Part model, mm, in its own coordinate system. A direction names the side the tool comes from. Round coordinates to 2 decimals unless told otherwise and drop trailing zeros. Write each loop counter-clockwise with the first axis right and the second up, starting at its lowest first coordinate (ties: lowest second). Pieces come first, ordered by that corner, then holes. Notation, with made-up numbers: M 30,-18 L 48,-18 A17 cw 48,-6 Z; hole C 44.25,59.5 d5. An arc over 180 degrees is marked long. Use a Markdown table: item, result. Add a question column.
1) Slice it at B-B on z = 59.5. Write the cut outline in (x, y), plus the area to 3 significant figures.
2) Two-plate mould, pull along X, no slides. Class faces 3 (the face through (-7, 18, 0)), 4 (the face through (-500, -18, 49)), 5 (the face through (500, 18, 49)), 6 (the face through (-416, 18, 100)): released by +X, released by -X, zero draft, split by the parting line, or undercut.
3) Which spindle directions (+Z, -Z, +X, -X, +Y, -Y) get a long thin tool onto all of the face, cutting with end or side? Do faces 1 (the face through (331, 18, 100)), 2 (the face through (77, -1300, 53)). Say none if no direction does.
4) Slice it at C-C on x = -426.5. Write the cut outline in (y, z).
5) Drop flat-ended pins along their axis: P1, Ø4, axis at x = 28.5, y = 896, coming from the -Z side; P2, Ø2, axis at x = -5.5, y = 582, coming from the +Z side; P3, Ø5, axis at y = 63.5, z = 106.5, coming from the +X side; P4, Ø12, axis at x = 215.5, y = -258.5, coming from the +Z side. Give the stop position or say it passes through.
6) Slice it at A-A on y = 389. Write the cut outline in (x, z).
7) Wall check: probe 1 along X at (y, z) = (-9, 125); probe 2 along X at (y, z) = (606, 11); probe 3 along X at (y, z) = (547, 133.5). Give the ranges that are in metal, low to high.
Autodesk Inventor part; units mm, degrees
ref_plane "YZ Plane" through (0, 0, 0) normal (1, 0, 0) x (0, 1, 0)
ref_plane "XZ Plane" through (0, 0, 0) normal (0, 1, 0) x (-1, 0, 0)
ref_plane "XY Plane" through (0, 0, 0) normal (0, 0, 1) x (1, 0, 0)
sketch "Sketch1" plane through (0, 0, 0) normal (0, 0, 1) x (1, 0, 0)
  line L0 (-500, 1300) -> (500, 1300)
  line L1 (500, 1300) -> (500, -1300)
  line L2 (500, -1300) -> (-500, -1300)
  line L3 (-500, -1300) -> (-500, 1300)
  line L4 (-500, 1300) -> (500, -1300) construction
  line L5 (500, 1300) -> (-500, -1300) construction
  point P0 (0, 0)
  dimension "d0" = 1000
  dimension "d1" = 2600
extrude "Extrusion1" add sketch "Sketch1" along normal blind 100
sketch "Sketch2" plane through (-500, -1300, 0) normal (0, -1, 0) x (1, 0, 0)
  line L0 (0, 0) -> (1000, 0)
  line L1 (1000, 0) -> (1000, 100)
  line L2 (0, 100) -> (1000, 100)
  line L3 (0, 0) -> (0, 100)
  line L4 (0, 100) -> (1000, 100)
  line L5 (1000, 100) -> (977, 135)
  line L6 (977, 135) -> (937, 135)
  line L7 (937, 135) -> (914, 100)
  line L8 (687, 135) -> (664, 100)
  line L9 (727, 135) -> (687, 135)
  line L10 (750, 100) -> (727, 135)
  line L11 (437, 135) -> (414, 100)
  line L12 (477, 135) -> (437, 135)
  line L13 (500, 100) -> (477, 135)
  line L14 (187, 135) -> (164, 100)
  line L15 (227, 135) -> (187, 135)
  line L16 (250, 100) -> (227, 135)
  line L17 (-63, 135) -> (-86, 100)
  line L18 (-23, 135) -> (-63, 135)
  line L19 (0, 100) -> (-23, 135)
  line L20 (-90.1785, 102.7459) -> (-65.6973, 140)
  line L21 (-65.6973, 140) -> (-20.3027, 140)
  line L22 (-20.3027, 140) -> (5.983, 100)
  line L23 (-90.1785, 102.7459) -> (-86, 100)
  point P0 (500, 0)
  point P1 (5.983, 100)
  dimension "d4" = 86
  dimension "d5" = 40
  dimension "d6" = 35
  dimension "d11" = 250
  dimension "d16" = 5
  dimension "d17" = 5
extrude "Extrusion2" add sketch "Sketch2" against normal up to surface (2600 mm away) contours L19 L18 L17 L23 L20 L21 L22 L2 | L2 L7 L6 L5 | L14 L15 L16 L2 | L2 L8 L9 L10 | L11 L12 L13 L2
chamfer "Chamfer1" distance 10 angle 45 2 edges at (500, -1300, 50) (500, 1300, 50)
equation "\"d17\" = d16"
properties part number "Sandwich 5  roof long"
Entries:
| question | item | result |
|---|---|---|
| 1 | outline | M -500,-1300 L 490,-1300 L 500,-1290 L 500,1290 L 490,1300 L -500,1300 Z |
| 1 | area | 2,600,000 mm^2 |
| 2 | face 3 | zero draft |
| 2 | face 4 | released by -X |
| 2 | face 5 | released by +X |
| 2 | face 6 | undercut |
| 3 | face 1 | +Z, +Y, -Y |
| 3 | face 2 | +Z, -Z, +X, -X, -Y |
| 4 | outline | M -1300,0 L 1300,0 L 1300,100 L -1300,100 Z |
| 5 | P1 | stops at z = 0 |
| 5 | P2 | stops at z = 109.89 |
| 5 | P3 | stops at x = 497.37 |
| 5 | P4 | stops at z = 135 |
| 6 | outline | M -590.18,102.75 L -586,100 L -563,135 L -523,135 L -500,100 L -500,0 L 500,0 L 500,100 L 477,135 L 437,135 L 414,100 L 250,100 L 227,135 L 187,135 L 164,100 L 0,100 L -23,135 L -63,135 L -86,100 L -250,100 L -273,135 L -313,135 L -336,100 L -494.02,100 L -520.3,140 L -565.7,140 Z |
| 7 | probe 1 | x = -575.55 to -569.57, -516.43 to -510.45, -319.57 to -266.43, -69.57 to -16.43, 180.43 to 233.57, 430.43 to 483.57 |
| 7 | probe 2 | x = -500 to 500 |
| 7 | probe 3 | x = -569.97 to -563.99, -522.01 to -516.03, -313.99 to -272.01, -63.99 to -22.01, 186.01 to 227.99, 436.01 to 477.99 |
